from build123d import *

# Parameters (mm, degrees)
F0_W     = 127
F0_H     = 88.9
F1_DEPTH = 50.8
F3_DEPTH = 25.4
F4_R     = 25.4
F5_DEPTH = 50.8


with BuildPart() as f1:
    # F0 (on Front) → F1 (new body)
    with BuildSketch(Plane.XZ):
        with Locations((63.5, -44.45)):
            Rectangle(F0_W, F0_H)
    extrude(amount=F1_DEPTH)

    # F2 (on face) → F3 (cut)
    with BuildSketch(Plane.XZ.offset(50.8)):
        Polygon((127, 0), (38.1, 0), (101.6, -88.9), (127, -88.9), align=None)
    extrude(amount=-F3_DEPTH, mode=Mode.SUBTRACT)

    # F4 (on face) → F5 (cut)
    with BuildSketch(Plane.XZ.offset(50.8)):
        with Locations((50.8, -38.1)):
            Circle(F4_R)
    extrude(amount=-F5_DEPTH, mode=Mode.SUBTRACT)


solid = f1.part
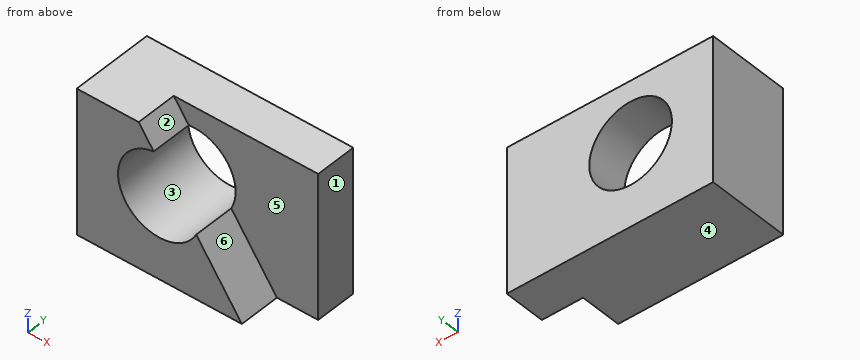
Model file for the job. Use its own axes, mm. Face numbers are marked on the shaded views. A direction names the side the tool comes from. Give positions to 0.01 mm unless a question says otherwise; leave off trailing zeros. Loops run counter-clockwise (first coordinate to the right, second up) from the corner with the lowest first, then second, coordinate; pieces in that order, holes last.
Item 1: Drop flat-ended pins along their axis: P1, Ø3, axis at y = -28.5, z = -52, coming from the +X side; P2, Ø3, axis at y = -31, z = -50, coming from the +X side; P3, Ø3, axis at x = 94.5, z = -16.5, coming from the -Y side. Give the stop position or say it passes through.
Check values:
P1: stops at x = 76.31
P2: stops at x = 74.89
P3: stops at y = -25.4
Item 2: Drill centre lines: line 1 along Z through (x, y) = (50, -22); line 2 along X through (y, z) = (-23.5, -38.1); line 3 along Y through (x, z) = (106.5, -84). Where is each one in solid material? Low to high.
Check values:
line 1: z = -88.9 to -63.49, -12.71 to 0
line 2: x = 0 to 25.4, 76.2 to 127
line 3: y = -25.4 to 0
Item 3: Slice it at D-D (y = -40.5). Write the cut outline in (x, z), plus the area to 3 significant figures.
Check values:
outline: (0, -88.9) - (101.6, -88.9) - (73.48, -49.53) arc R25.4 cw (long way) to (47.34, -12.94) - (38.1, 0) - (0, 0) - close
area: 4,620 mm2
Item 4: Slice it at C-C (y = -7). Write the cut outline in (x, z).
Check values:
outline: (0, -88.9) - (127, -88.9) - (127, 0) - (0, 0) - close; hole circle Ø50.8 at (50.8, -38.1)
Item 5: Slice it at A-A (x = 50.8). Write the cut outline in (y, z), plus the area to 3 significant figures.
Check values:
outline: (-50.8, -88.9) - (0, -88.9) - (0, -63.5) - (-50.8, -63.5) - close; (-25.4, -12.7) - (0, -12.7) - (0, 0) - (-25.4, 0) - close
area: 1,610 mm2
Item 6: Mould opens along Z. For the marked faces 3, 4, 5 and 6 say: +Z half, -Z half, draft (parallel to the pull), parting line (faces both ways), or undercut.
Check values:
face 3: undercut
face 4: -Z half
face 5: draft
face 6: +Z half
Item 7: Which spindle directions (+Z, -Z, +X, -X, +Y, -Y) get a long thin tool onto all of the face, cutting with end or side? Do the marked faces 1 and 2. Say none if no direction does.
Check values:
face 1: +Z, -Z, +X, +Y, -Y
face 2: +Z, +X, -Y
Item 8: Slice it at B-B (z = -38.1). Write the cut outline in (x, y).
Check values:
outline: (0, -50.8) - (25.4, -50.8) - (25.4, 0) - (0, 0) - close; (76.2, -25.4) - (127, -25.4) - (127, 0) - (76.2, 0) - close
